Check sheet for the modelled part. Datum: model origin and axes. Units: mm. Face numbers are marked on the shaded views. A direction names the side the tool comes from. Round coordinates to 2 decimals unless told otherwise and drop trailing zeros. Order: outer loops, then holes, each group sorted by start corner. A loop starts at its lowest first (then second) coordinate and runs counter-clockwise, first axis right, second up. Notation, with made-up numbers: M 15.25,-28 L 55.25,-28 A33 ccw 55.25,11 Z; hole C 14.25,24 d6. An arc over 180 degrees is marked long. One line per item, written item: value. Start each with the question number.
(1) Depth check by flat-ended pin: pin 1 Ø5 at (y, z) = (4, -3.5) entering from +X; pin 2 Ø5 at (x, z) = (1.5, -1) entering from +Y. Enter the tip coordinate at first touch or a pass-through.
(2) Cross-section at B-B, the plane z = 0. Enter the section's corners in (x, y).
(3) Cross-section at D-D, the plane z = 3.25. Enter the section's corners in (x, y).
(4) Release check for a two-part mould opening along Z. For the marked faces 1, 2 and 3 record: released by +Z, released by -Z, zero draft, split by the parting line, or undercut.
(5) Cross-section at C-C, the plane x = 0. Enter the section's corners in (y, z), and give its area (3 significant figures).
(6) Cross-section at A-A, the plane y = 2.35. Enter the section's corners in (x, z), and give its area (3 significant figures).
(7) Thickness scan on L1, parallel to Z at x = 0, y = -4.9; L2, parallel to Y at x = -3.6, z = 0. Record the ranges inside material, lowest first.
(8) Access from +Z, -Z, +X, -X, +Y, -Y to the whole of each face (thin tool, end or side, straight path). Record for the marked faces 4 and 5.
from build123d import *

# Parameters (mm, degrees)
BOSS_EXTRUDE1_DEPTH = 5
SKETCH2_R           = 1.65
CUT_EXTRUDE1_DEPTH  = 3
SKETCH3_R           = 1.65
CUT_EXTRUDE2_DEPTH  = 10


with BuildPart() as part:
    # Sketch1 → Boss-Extrude1 (new body, symmetric)
    with BuildSketch(Plane.XY):
        Polygon((-5, 6.35), (-5, -6.35), (5, -6.35), (5, -4.35), (-3, -4.35), (-3, 6.35), align=None)
    extrude(amount=BOSS_EXTRUDE1_DEPTH, both=True)

    # Sketch2 → Cut-Extrude1 (cut, through all)
    with BuildSketch(Plane(origin=(0, -4.35, 0), x_dir=(1, 0, 0), z_dir=(0, 1, 0))):
        Circle(SKETCH2_R)
    extrude(amount=-CUT_EXTRUDE1_DEPTH, mode=Mode.SUBTRACT)

    # Sketch3 → Cut-Extrude2 (cut)
    with BuildSketch(Plane(origin=(-3, 0, 0), x_dir=(0, 0, -1), z_dir=(1, 0, 0))):
        with Locations((0, 2.35)):
            Circle(SKETCH3_R)
    extrude(amount=-CUT_EXTRUDE2_DEPTH, mode=Mode.SUBTRACT)


solid = part.part
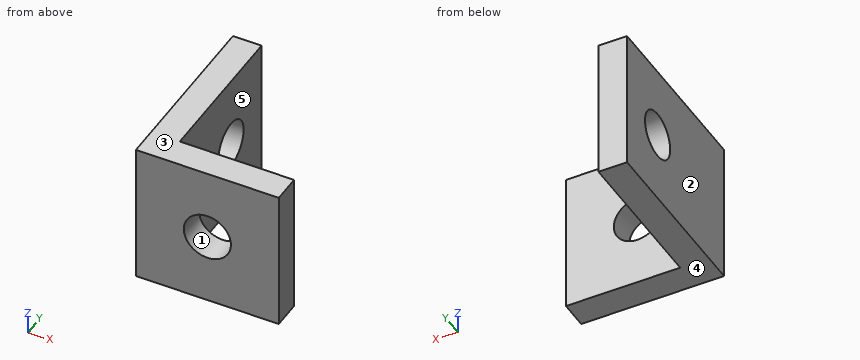
Values found:
1. pin 1: x = -3
1. pin 2: y = -4.35
2. outline: M -5,-6.35 L -1.65,-6.35 L -1.65,-4.35 L -3,-4.35 L -3,0.7 L -5,0.7 Z; M -5,4 L -3,4 L -3,6.35 L -5,6.35 Z; M 1.65,-6.35 L 5,-6.35 L 5,-4.35 L 1.65,-4.35 Z
3. outline: M -5,-6.35 L 5,-6.35 L 5,-4.35 L -3,-4.35 L -3,6.35 L -5,6.35 Z
4. face 1: undercut
4. face 2: zero draft
4. face 3: released by +Z
5. outline: M -6.35,-5 L -4.35,-5 L -4.35,-1.65 L -6.35,-1.65 Z; M -6.35,1.65 L -4.35,1.65 L -4.35,5 L -6.35,5 Z
5. area: 13.4 mm^2
6. outline: M -5,-5 L -3,-5 L -3,-1.65 L -5,-1.65 Z; M -5,1.65 L -3,1.65 L -3,5 L -5,5 Z
6. area: 13.4 mm^2
7. L1: -5 to -1.65, 1.65 to 5
7. L2: -6.35 to 0.7, 4 to 6.35
8. face 4: -Z, +X, -X, +Y, -Y
8. face 5: +Z, -Z, +X, +Y
